```python
from build123d import *
from OCP.BRepAlgoAPI import BRepAlgoAPI_Cut
from OCP.TopTools import TopTools_ListOfShape

# Parameters (mm, degrees)
SKETCH_1_R          = 6
SKETCH_1_R_2        = 4
EXTRUDE_1_DEPTH     = 25
CUT_EXTRUDE_START   = -17
SKETCH_3_R          = 4
CUT_EXTRUDE_2_DEPTH = 17


with BuildPart() as part:
    # 草图1 → 凸台-拉伸1 (new body)
    with BuildSketch(Plane.XY):
        Circle(SKETCH_1_R)
        Circle(SKETCH_1_R_2, mode=Mode.SUBTRACT)
    extrude(amount=EXTRUDE_1_DEPTH)

    # 草图2 → 旋转3 (revolve)
    with BuildSketch(Plane(origin=(0, 0, 0), x_dir=(1, 0, 0), z_dir=(0, 1, 0))):
        with BuildLine():
            Line((0, 10), (0, -10))
            ThreePointArc((0, -10), (-10, 0), (0, 10))
        make_face()
    revolve(axis=Axis((0, 0, 0), (0, 0, -1)))

    # 草图3 → 切除-拉伸2 (cut)
    with BuildSketch(Plane.XY.offset(25).offset(CUT_EXTRUDE_START)):
        Circle(SKETCH_3_R)
    extrude(amount=CUT_EXTRUDE_2_DEPTH, mode=Mode.SUBTRACT)


with BuildPart() as cut_revolve_1_tool:
    # 草图4 → 切除-旋转1 (revolve)
    with BuildSketch(Plane(origin=(0, 0, 0), x_dir=(0, 0, -1), z_dir=(1, 0, 0))):
        with BuildLine():
            Line((0, 7), (0, -7))
            Line((0, -7), (0, -10))
            Line((0, -10), (6, -10))
            Line((6, -10), (7.857142857, -6.185895741))
            Line((7.857142857, -6.185895741), (5.5, -4.330127019))
            ThreePointArc((5.5, -4.330127019), (6.297256908, 3.056886559), (0, 7))
        make_face()
    revolve(axis=Axis((0, 0, 0), (0, 1, 0)))


with BuildPart() as part_1:
    add(part.part)

    # 切除-旋转1: cut by cut_revolve_1_tool, with a tolerance
    cut_revolve_1_stock = TopTools_ListOfShape()
    cut_revolve_1_stock.Append(part_1.part.wrapped)
    cut_revolve_1_tools = TopTools_ListOfShape()
    cut_revolve_1_tools.Append(cut_revolve_1_tool.part.wrapped)
    cut_revolve_1_cut = BRepAlgoAPI_Cut()
    cut_revolve_1_cut.SetArguments(cut_revolve_1_stock)
    cut_revolve_1_cut.SetTools(cut_revolve_1_tools)
    cut_revolve_1_cut.SetFuzzyValue(0.00001)
    cut_revolve_1_cut.Build()
    add(Compound.cast(cut_revolve_1_cut.Shape()).solids(), mode=Mode.REPLACE)


solid = part_1.part
```
Work out the finished part from the listing and answer in its coordinate system (mm). Give positions to 0.01 mm unless a question says otherwise; leave off trailing zeros. Loops run counter-clockwise (first coordinate to the right, second up) from the corner with the lowest first, then second, coordinate; pieces in that order, holes last. Notation, with made-up numbers: (81.5, -4) -> (87.5, -4) arc R22 ccw to (87.5, 9) -> close; hole circle Ø4 at (52.5, -15.5). An arc over 180 degrees is marked (long way). One line per question, with ' | ' between items. Start each with the question number.
1) Section D-D, the plane y = 2 is taken. Determine the outline of the cut face in (x, z), then the cut area to 3 significant figures.
2) Straight lines are drawn through the part: L1, parallel to Y at x = 0, z = 21; L2, parallel to Z at x = -4.75, y = -3; L3, parallel to Z at x = -5.75, y = 2.75. For each, find the intervals that lie inside material, in ascending order.
3) Each of these flat-tipped pins is pushed along its axis until it touches: pin 1 (5 mm diameter, centred on x = 0, y = 6.5, fed in from -Z); pin 2 (1.5 mm diameter, centred on x = -1.5, y = 0, fed in from -Z); pin 3 (12 mm diameter, centred on x = -6.5, z = 6, fed in from +Y). Where does it stop, or does it pass through?
4) Section C-C, the plane z = 9 is taken. Determine the outline of the cut face in (x, y).
5) Section A-A, the plane y = 0 is taken. Determine the outline of the cut face in (x, z), then the cut area to 3 significant figures.
6) Determine the mould class of faces 1 (the face through (-6, 0, 16)), 2 (the face through (-0.867, -3.905, 16.381)), 3 (the face through (-1.42, -3.92, 25)) for opening direction X: +X half, -X half, draft (parallel to the pull), parting line (faces both ways), or undercut.
Resolved:
1) outline: (-5.66, 8) arc R9.8 ccw (long way) to (5.66, 8) -> (5.66, 25) -> (3.46, 25) -> (3.46, 8) -> (-3.46, 8) -> (-3.46, 25) -> (-5.66, 25) -> close; hole circle Ø13.42 at (0, 0) | area: 221 mm2
2) L1: -6 to -4, 4 to 6 | L2: -8.27 to -4.18, 4.18 to 25 | L3: -7.71 to -2.89, 2.89 to 7.71
3) pin 1: z = -9.17 | pin 2: z = -9.97 | pin 3: y = 9.59
4) outline: circle Ø12 at (0, 0); hole circle Ø8 at (0, 0)
5) outline: (-6, 8) arc R10 ccw (long way) to (6, 8) -> (6, 25) -> (4, 25) -> (4, 8) -> (-4, 8) -> (-4, 25) -> (-6, 25) -> close; hole circle Ø14 at (0, 0) | area: 212 mm2
6) face 1: parting line | face 2: undercut | face 3: draft
